Source: CAD feature listing. Evaluate the final solid. Frame: model axes, mm. Face numbers are marked on the shaded views. Give positions to 0.01 mm unless a question says otherwise; leave off trailing zeros. Loops run counter-clockwise (first coordinate to the right, second up) from the corner with the lowest first, then second, coordinate; pieces in that order, holes last. Notation, with made-up numbers: (33.25, -4.75) -> (92.25, -4.75) arc R27 ccw to (92.25, 28.25) -> close; hole circle Ø1 at (65.5, 3). An arc over 180 degrees is marked (long way). Put each result on its own line as item: value.
```python
from build123d import *

# Parameters (mm, degrees)
SKETCH1_W               = 86
SKETCH1_H               = 28.2
BOSS_EXTRUDE1_DEPTH     = 2
SKETCH5_R               = 1.05
BOSS_EXTRUDE2_DEPTH     = 5
SKETCH8_W               = 1.75956426
SKETCH8_H               = 1.75956426
CUT_EXTRUDE3_DEPTH      = 5
FILLET4_R               = 0.2
LPATTERN1_COUNT         = 12
LPATTERN1_PITCH         = 5
LPATTERN1_2_COUNT       = 12
LPATTERN1_2_PITCH       = 5
FILLET4_OF_LPATTERN1_R  = 0.2
CUT_EXTRUDE1_START      = -43
CUT_EXTRUDE1_DEPTH      = 5
FILLET5_R               = 1.5
BOSS_EXTRUDE3_DEPTH     = 1
CUT_EXTRUDE6_DEPTH      = 47.407525329
CUT_EXTRUDE6_DEPTH_BACK = 47.407525329
SKETCH10_W              = 7
SKETCH10_H              = 15
FILLET6_R               = 2


# Read off the part's stored shape, not the designer's step: Cut-Extrude1
with BuildPart() as part:
    # Sketch1 → Boss-Extrude1 (new body)
    with BuildSketch(Plane.XY):
        Rectangle(SKETCH1_W, SKETCH1_H)
    extrude(amount=BOSS_EXTRUDE1_DEPTH)


with BuildPart() as body_2:
    # Sketch5 → Boss-Extrude2 (new body)
    with BuildSketch(Plane.ZY.offset(43)):
        with BuildLine():
            Line((0.5, 15.6), (0, 14.1))
            Line((0, 14.1), (2, 14.1))
            ThreePointArc((2, 14.1), (3.060660172, 16.660660172), (0.5, 15.6))
        make_face()
        with Locations((2, 15.6)):
            Circle(SKETCH5_R, mode=Mode.SUBTRACT)
    boss_extrude2 = extrude(amount=-BOSS_EXTRUDE2_DEPTH)

    # Sketch8 → Cut-Extrude3 (cut)
    with BuildSketch(Plane.ZY.offset(43)):
        with Locations((3.068777943, 16.78020761)):
            Rectangle(SKETCH8_W, SKETCH8_H)
    cut_extrude3 = extrude(amount=-CUT_EXTRUDE3_DEPTH, mode=Mode.SUBTRACT)

    # Fillet4
    fillet4_edges = [body_2.edges().sort_by_distance(p)[0] for p in [
        (-40.5, 16.632850707, 2.188995813),
        (-40.5, 15.90042548, 3.006103638),
        (-40.5, 17.088045894, 2.188995813),
        (-40.5, 15.90042548, 3.469606931),
    ]]
    fillet(fillet4_edges, radius=FILLET4_R)


with BuildPart() as part_1:
    add(part.part)

    add(body_2.part)  # LPattern1 merges body 2
    # LPattern1: Boss-Extrude2 ×12, 5 skipped
    with Locations(*[(i * LPATTERN1_PITCH, 0, 0) for i in range(1, LPATTERN1_COUNT) if i not in (2, 4, 6, 8, 10)]):
        add(boss_extrude2)

    # LPattern1 2: Cut-Extrude3 ×12, 5 skipped
    with Locations(*[(i * LPATTERN1_2_PITCH, 0, 0) for i in range(1, LPATTERN1_2_COUNT) if i not in (2, 4, 6, 8, 10)]):
        add(cut_extrude3, mode=Mode.SUBTRACT)

    # Fillet4 of LPattern1
    fillet4_of_lpattern1_edges = [part_1.edges().sort_by_distance(p)[0] for p in [
        (-35.5, 16.632850707, 2.188995813),
        (-35.5, 15.90042548, 3.006103638),
        (-35.5, 17.088045894, 2.188995813),
        (-35.5, 15.90042548, 3.469606931),
        (-25.5, 16.632850707, 2.188995813),
        (-25.5, 15.90042548, 3.006103638),
        (-25.5, 17.088045894, 2.188995813),
        (-25.5, 15.90042548, 3.469606931),
        (-15.5, 16.632850707, 2.188995813),
        (-15.5, 15.90042548, 3.006103638),
        (-15.5, 17.088045894, 2.188995813),
        (-15.5, 15.90042548, 3.469606931),
        (-5.5, 16.632850707, 2.188995813),
        (-5.5, 15.90042548, 3.006103638),
        (-5.5, 17.088045894, 2.188995813),
        (-5.5, 15.90042548, 3.469606931),
        (4.5, 16.632850707, 2.188995813),
        (4.5, 15.90042548, 3.006103638),
        (4.5, 17.088045894, 2.188995813),
        (4.5, 15.90042548, 3.469606931),
        (14.5, 16.632850707, 2.188995813),
        (14.5, 15.90042548, 3.006103638),
        (14.5, 17.088045894, 2.188995813),
        (14.5, 15.90042548, 3.469606931),
    ]]
    fillet(fillet4_of_lpattern1_edges, radius=FILLET4_OF_LPATTERN1_R)

    # Cut-Extrude1 outline → Cut-Extrude1 (cut)
    with BuildSketch(Plane.YZ.offset(CUT_EXTRUDE1_START)):
        with BuildLine():
            Line((14.1, 2), (14.1, 0))
            Line((14.1, 0), (15.6, 0.5))
            ThreePointArc((15.6, 0.5), (16.656161515, 0.934860171), (17.09994626, 1.987302861))
            ThreePointArc((17.09994626, 1.987302861), (17.041972069, 2.129817348), (16.899953425, 2.188995813))
            Line((16.899953425, 2.188995813), (16.849951562, 2.188995813))
            ThreePointArc((16.849951562, 2.188995813), (16.709154073, 2.131038296), (16.649959312, 1.990756483))
            ThreePointArc((16.649959312, 1.990756483), (14.825162546, 1.291390855), (15.684357403, 3.046605861))
            ThreePointArc((15.684357403, 3.046605861), (15.836046984, 3.098966816), (15.90042548, 3.245959359))
            Line((15.90042548, 3.245959359), (15.90042548, 3.296115243))
            ThreePointArc((15.90042548, 3.296115243), (15.847207656, 3.431964397), (15.715875553, 3.495517588))
            ThreePointArc((15.715875553, 3.495517588), (14.581131346, 3.100866325), (14.1, 2))
        make_face()
    extrude(amount=CUT_EXTRUDE1_DEPTH, mode=Mode.SUBTRACT)

    # Fillet5
    fillet5_edges = [part_1.edges().sort_by_distance(p)[0] for p in [
        (0, -14.1, 0),
        (-43, 0, 0),
        (43, 0, 0),
    ]]
    fillet(fillet5_edges, radius=FILLET5_R)

    # Sketch9 → Boss-Extrude3 (add)
    with BuildSketch(Plane.XY.offset(2)):
        Polygon((-41.7, 11.6), (-40.7, 11.6), (-40.7, -11.85), (40.7, -11.85), (40.7, 11.6), (41.7, 11.6), (41.7, -11.85), (41.7, -12.85), (-40.7, -12.85), (-41.7, -12.85), align=None)
    extrude(amount=BOSS_EXTRUDE3_DEPTH)

    # Sketch10 → Cut-Extrude6 (cut, two sides: drawn at the far end of the back side and taken through both)
    with BuildSketch(Plane(origin=(0, 0, 0), x_dir=(-1, 0, 0), z_dir=(0, 0, -1)).offset(-CUT_EXTRUDE6_DEPTH_BACK)):
        with Locations((-31.5, 0.75)):
            Rectangle(SKETCH10_W, SKETCH10_H)
    extrude(amount=CUT_EXTRUDE6_DEPTH + CUT_EXTRUDE6_DEPTH_BACK, mode=Mode.SUBTRACT)

    # Fillet6
    fillet6_edges = [part_1.edges().sort_by_distance(p)[0] for p in [
        (28, -6.75, 1),
        (28, 8.25, 1),
        (35, 8.25, 1),
        (35, -6.75, 1),
    ]]
    fillet(fillet6_edges, radius=FILLET6_R)


solid = part_1.part
```
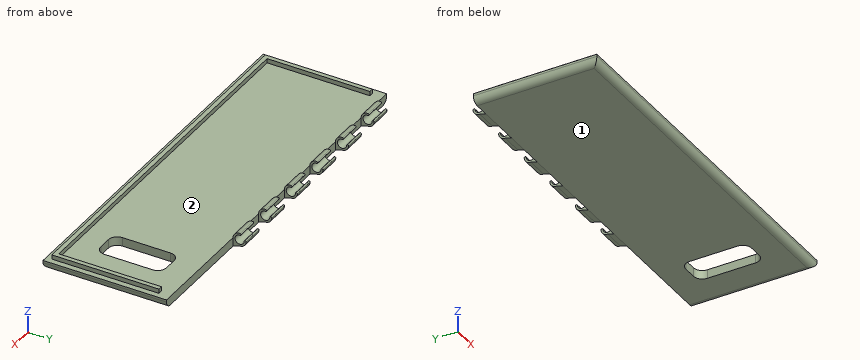
(1) Line query: probe 1 along X at (y, z) = (-5, 2.45); probe 2 along Y at (x, z) = (14.5, 2.1); probe 3 along X at (y, z) = (15, 1.1). Output: solid intervals per line, ascending. Write a range as from..to.
Calculated:
probe 1: x = -41.7..-40.7, 40.7..41.7
probe 2: y = -12.85..-11.85, 14.1..14.55, 16.68..17.07
probe 3: x = -38..-33, -28..-23, -18..-13, -8..-3, 2..7, 12..17
(2) Draft query along X for the marked faces 1 and 2. Return one class per face: released by +X, released by -X, zero draft, split by the parting line, or undercut.
Calculated:
face 1: zero draft
face 2: undercut
(3) Section B-B on y = -11. Return loops of the section in (x, z).
Calculated:
outline: (-43, 1.5) arc R1.5 ccw to (-41.5, 0) -> (41.5, 0) arc R1.5 ccw to (43, 1.5) -> (43, 2) -> (41.7, 2) -> (41.7, 3) -> (40.7, 3) -> (40.7, 2) -> (-40.7, 2) -> (-40.7, 3) -> (-41.7, 3) -> (-41.7, 2) -> (-43, 2) -> close
(4) Section C-C on y = 13. Return loops of the section in (x, z), then the cut area to 3 significant figures.
Calculated:
outline: (-43, 1.5) arc R1.5 ccw to (-41.5, 0) -> (41.5, 0) arc R1.5 ccw to (43, 1.5) -> (43, 2) -> (-43, 2) -> close
area: 171 mm²
(5) Section A-A on x = -11.5. Return loops of the section in (y, z).
Calculated:
outline: (-14.1, 1.5) arc R1.5 ccw to (-12.6, 0) -> (14.1, 0) -> (14.1, 2) -> (-11.85, 2) -> (-11.85, 3) -> (-12.85, 3) -> (-12.85, 2) -> (-14.1, 2) -> close
(6) First-contact query: P1, Ø1.1, axis at x = -9.5, z = 2.5, coming from the +Y side; P2, Ø1.5, axis at x = -20.5, y = -5, coming from the +Z side; P3, Ø0.8, axis at y = 1, z = 2.5, coming from the +X side; P4, Ø6, axis at x = -3.5, y = 14, coming from the +Z side. Flat tips, straight axial feed; report the tip coordinate or a pass-through.
Calculated:
P1: stops at y = 14.1
P2: stops at z = 2
P3: stops at x = 41.7
P4: stops at z = 3.5
